Check sheet for the modelled part. Datum: model origin and axes. Units: mm. A direction names the side the tool comes from. Round coordinates to 2 decimals unless told otherwise and drop trailing zeros. Write each loop counter-clockwise with the first axis right and the second up, starting at its lowest first coordinate (ties: lowest second). Pieces come first, ordered by that corner, then holes. Notation, with made-up numbers: (-13.75, 20.25) -> (0.25, 20.25) arc R19 ccw to (0.25, 49.25) -> close; hole circle Ø5 at (58, 64). An arc over 180 degrees is marked (long way). One line per item, written item: value.
from build123d import *

# Parameters (mm, degrees)
SKETCH_1_W          = 40
SKETCH_1_H          = 7
EXTRUDE_1_DEPTH     = 3
SKETCH_2_W          = 26
SKETCH_2_H          = 7
EXTRUDE_2_DEPTH     = 62
SKETCH_3_R          = 7.8
CUT_EXTRUDE_1_DEPTH = 7
SKETCH_4_R          = 1.5
CUT_EXTRUDE_2_DEPTH = 7
SKETCH_5_R          = 1.5
CUT_EXTRUDE_3_DEPTH = 7


with BuildPart() as part:
    # Эскиз1 → Бобышка-Вытянуть1 (new body)
    with BuildSketch(Plane.XY):
        Rectangle(SKETCH_1_W, SKETCH_1_H)
    extrude(amount=EXTRUDE_1_DEPTH)

    # Эскиз2 → Бобышка-Вытянуть2 (add)
    with BuildSketch(Plane.XY.offset(3)):
        Rectangle(SKETCH_2_W, SKETCH_2_H)
    extrude(amount=EXTRUDE_2_DEPTH)

    # Эскиз3 → Вырез-Вытянуть1 (cut)
    with BuildSketch(Plane(origin=(0, -3.5, 0), x_dir=(-1, 0, 0), z_dir=(0, -1, 0))):
        with Locations((0, -50)):
            Circle(SKETCH_3_R)
    extrude(amount=-CUT_EXTRUDE_1_DEPTH, mode=Mode.SUBTRACT)

    # Эскиз4 → Вырез-Вытянуть2 (cut)
    with BuildSketch(Plane.XY.offset(3)):
        with Locations((-16.5, 0)):
            Circle(SKETCH_4_R)
    extrude(amount=-CUT_EXTRUDE_2_DEPTH, mode=Mode.SUBTRACT)

    # Эскиз5 → Вырез-Вытянуть3 (cut)
    with BuildSketch(Plane.XY.offset(3)):
        with Locations((16.5, 0)):
            Circle(SKETCH_5_R)
    extrude(amount=-CUT_EXTRUDE_3_DEPTH, mode=Mode.SUBTRACT)


solid = part.part
Item 1: Sectioned sample at A-A (x = 0). Enter the section's corners in (y, z).
Result set:
outline: (-3.5, 0) -> (3.5, 0) -> (3.5, 42.2) -> (-3.5, 42.2) -> close; (-3.5, 57.8) -> (3.5, 57.8) -> (3.5, 65) -> (-3.5, 65) -> close
Item 2: Material ranges on line 1 along Y through (x, z) = (16.5, 1.95); line 2 along X through (y, z) = (-0.25, 50); line 3 along Z through (x, y) = (0, 2), recorded low to high.
Result set:
line 1: -3.5 to -1.5, 1.5 to 3.5
line 2: -13 to -7.8, 7.8 to 13
line 3: 0 to 42.2, 57.8 to 65
Item 3: Release check for a two-part mould opening along X. For faces 4 (the cylindrical face through (15, 0, 2)), 5 (the flat face through (0, -3.5, 32)), 6 (the flat face through (-13, 0, 34)) record: pulls with the +X half, pulls with the -X half, needs draft (parallel to the pull), parting line crosses it, or undercut.
Result set:
face 4: undercut
face 5: needs draft
face 6: pulls with the -X half
Item 4: Sectioned sample at C-C (z = 50). Enter the section's corners in (x, y), then the cut area to 3 significant figures.
Result set:
outline: (-13, -3.5) -> (-7.8, -3.5) -> (-7.8, 3.5) -> (-13, 3.5) -> close; (7.8, -3.5) -> (13, -3.5) -> (13, 3.5) -> (7.8, 3.5) -> close
area: 72.8 mm^2
Item 5: Tool access check on faces 1 (the flat face through (-17, -2, 3)), 2 (the flat face through (16, -2, 3)), 3 (the cylindrical face through (1.691, -0.049, 57.615)). Record the directions out of +Z, -Z, +X, -X, +Y, -Y that give a thin tool (end or side, any length) a straight path to the whole face; none if there is none.
Result set:
face 1: +Z, -X, +Y, -Y
face 2: +Z, +X, +Y, -Y
face 3: +Y, -Y
Item 6: Sectioned sample at D-D (z = 22.5). Enter the section's corners in (x, y).
Result set:
outline: (-13, -3.5) -> (13, -3.5) -> (13, 3.5) -> (-13, 3.5) -> close
Item 7: Depth check by flat-ended pin: pin 1 (20.5 mm diameter, centred on x = 0, z = 50, fed in from +Y); pin 2 (2 mm diameter, centred on x = 17.5, y = 0.5, fed in from +Z); pin 3 (3 mm diameter, centred on y = -2.5, z = 45.5, fed in from -X); pin 4 (2 mm diameter, centred on y = 0, z = 45, fed in from +X). Enter the tip coordinate at first touch or a pass-through.
Result set:
pin 1: y = 3.5
pin 2: z = 3
pin 3: x = -13
pin 4: x = 13
Item 8: Sectioned sample at B-B (y = 0). Enter the section's corners in (x, z), then the cut area to 3 significant figures.
Result set:
outline: (-20, 0) -> (-18, 0) -> (-18, 3) -> (-20, 3) -> close; (-15, 0) -> (15, 0) -> (15, 3) -> (13, 3) -> (13, 65) -> (-13, 65) -> (-13, 3) -> (-15, 3) -> close; (18, 0) -> (20, 0) -> (20, 3) -> (18, 3) -> close; hole circle Ø15.6 at (0, 50)
area: 1,520 mm^2
